from build123d import *

# Parameters (mm, degrees)
CYLINDER_R           = 1.25
CYLINDER_DEPTH       = 2
CYLINDER_PITCH_ANGLE = 90
ARRAY_X_COUNT        = 2
ARRAY_X_PITCH        = 38
ARRAY_Y_COUNT        = 2
ARRAY_Y_PITCH        = 27.5
CYLINDER001_R        = 2
CYLINDER001_DEPTH    = 2
ARRAY001_X_COUNT     = 2
ARRAY001_X_PITCH     = 22
ARRAY001_Y_COUNT     = 2
ARRAY001_Y_PITCH     = 40
BOX001_W             = 2
BOX001_H             = 60
BOX001_DEPTH         = 20
BOX_W                = 40
BOX_H                = 60
BOX_DEPTH            = 2
BOX002_W             = 2
BOX002_H             = 60
BOX002_DEPTH         = 20


with BuildPart() as array:
    # Cylinder → Cylinder (new body)
    with BuildSketch(Plane.XY):
        Circle(CYLINDER_R)
    extrude(amount=CYLINDER_DEPTH)


with BuildPart() as array_1:
    # Cylinder pitch: moved
    add(array.part.rotate(Axis((0, 0, 0), (0, 1, 0)), CYLINDER_PITCH_ANGLE))


with BuildPart() as array_2:
    # Cylinder placement: moved
    add(array_1.part.moved(Location((0, 16.4, 13.5))))

    # Array X: Array ×2


with BuildPart() as array_3:
    add(array_2.part)
    with Locations(*[(i * ARRAY_X_PITCH, 0, 0) for i in range(1, ARRAY_X_COUNT)]):
        add(array_2.part)

    # Array Y: Array ×2


with BuildPart() as array_4:
    add(array_3.part)
    with Locations(*[(0, i * ARRAY_Y_PITCH, 0) for i in range(1, ARRAY_Y_COUNT)]):
        add(array_3.part)


with BuildPart() as array_5:
    # Array placement: moved
    add(array_4.part.moved(Location((2, 40, 0))))


with BuildPart() as array001:
    # Cylinder001 → Cylinder001 (new body)
    with BuildSketch(Plane(origin=(11, 48, 0), x_dir=(1, 0, 0), z_dir=(0, 0, 1))):
        Circle(CYLINDER001_R)
    extrude(amount=CYLINDER001_DEPTH)

    # Array001 X: Array001 ×2


with BuildPart() as array001_1:
    add(array001.part)
    with Locations(*[(i * ARRAY001_X_PITCH, 0, 0) for i in range(1, ARRAY001_X_COUNT)]):
        add(array001.part)

    # Array001 Y: Array001 ×2


with BuildPart() as array001_2:
    add(array001_1.part)
    with Locations(*[(0, i * ARRAY001_Y_PITCH, 0) for i in range(1, ARRAY001_Y_COUNT)]):
        add(array001_1.part)


with BuildPart() as cubo001:
    # Box001 → Box001 (new body)
    with BuildSketch(Plane.XY):
        with Locations((1, 30)):
            Rectangle(BOX001_W, BOX001_H)
    extrude(amount=BOX001_DEPTH)


with BuildPart() as cubo:
    # Box → Box (new body)
    with BuildSketch(Plane.XY):
        with Locations((20, 30)):
            Rectangle(BOX_W, BOX_H)
    extrude(amount=BOX_DEPTH)


with BuildPart() as cut002:
    # Box002 → Box002 (new body)
    with BuildSketch(Plane(origin=(38, 0, 0), x_dir=(1, 0, 0), z_dir=(0, 0, 1))):
        with Locations((1, 30)):
            Rectangle(BOX002_W, BOX002_H)
    extrude(amount=BOX002_DEPTH)

    # Fusion: union Cubo001, Cubo
    add(cubo001.part)
    add(cubo.part)

    # Cut: cut Array
    add(array_5.part, mode=Mode.SUBTRACT)


with BuildPart() as cut002_1:
    # Cut placement: moved
    add(cut002.part.moved(Location((2, 40, 0))))

    # Cut001: cut Array001
    add(array001_2.part, mode=Mode.SUBTRACT)

    # Cut002: cut Array
    add(array_5.part, mode=Mode.SUBTRACT)


solid = cut002_1.part
The listing builds one solid part. Answer for the finished solid, in the listing's coordinates (mm). A direction names the side the tool comes from. Coordinates: 2 decimals unless noted, no trailing zeros. Loops run counter-clockwise (first coordinate to the right, second up) from the corner with the lowest first, then second, coordinate; pieces in that order, holes last.
1) Find section A-A on y = 88. Write down the section's boundary in (x, z).
2) Find the intervals of material crossed by L1, parallel to Y at x = 33, z = 1.15; L2, parallel to X at y = 88, z = 0.7; L3, parallel to X at y = 59.5, z = 12.5, in increasing order.
3) Determine the mould class of faces 1 (the face through (2.99, 55.18, 13.77)), 2 (the face through (21.9, 40, 1.8)), 3 (the face through (3, 70, 20)), 4 (the face through (2.986, 82.791, 12.923)) for opening direction Z: pulls with the +Z half, pulls with the -Z half, needs draft (parallel to the pull), parting line crosses it, or undercut.
4) Find section D-D on y = 56.4. Write down the section's boundary in (x, z), then the cut area to 3 significant figures.
5) A tool of negligible diameter and unlimited length cuts with its end or side. For faces 5 (the face through (41, 70, 20)), 6 (the face through (40, 70, 11)), from which of +Z, -Z, +X, -X, +Y, -Y can it reach the whole face along a straight path? Write none if from no direction.
6) Flat-ended cylindrical pins translate along their axes: pin 1 Ø4.5 at (x, y) = (33, 48) entering from +Z; pin 2 Ø2 at (y, z) = (56.4, 13.5) entering from +X. Find the tip coordinate at first contact, or state that the pin passes through.
7) Find section C-C on x = 33. Write down the section's boundary in (y, z), then the cut area to 3 significant figures.
8) Find section B-B on z = 7.25. Write down the section's boundary in (x, y).
Values:
1. outline: (2, 0) - (9, 0) - (9, 2) - (4, 2) - (4, 20) - (2, 20) - close; (13, 0) - (31, 0) - (31, 2) - (13, 2) - close; (35, 0) - (42, 0) - (42, 20) - (40, 20) - (40, 2) - (35, 2) - close
2. L1: y = 40 to 46, 50 to 86, 90 to 100
2. L2: x = 2 to 9, 13 to 31, 35 to 42
2. L3: x = 2 to 4, 40 to 42
3. face 1: undercut
3. face 2: needs draft
3. face 3: pulls with the +Z half
3. face 4: undercut
4. outline: (2, 0) - (42, 0) - (42, 12.25) - (40, 12.25) - (40, 2) - (4, 2) - (4, 12.25) - (2, 12.25) - close; (2, 14.75) - (4, 14.75) - (4, 20) - (2, 20) - close; (40, 14.75) - (42, 14.75) - (42, 20) - (40, 20) - close
4. area: 142 mm2
5. face 5: +Z, +X, -X, +Y, -Y
5. face 6: +Z, +Y, -Y
6. pin 1: stops at z = 2
6. pin 2: passes through
7. outline: (40, 0) - (46, 0) - (46, 2) - (40, 2) - close; (50, 0) - (86, 0) - (86, 2) - (50, 2) - close; (90, 0) - (100, 0) - (100, 2) - (90, 2) - close
7. area: 104 mm2
8. outline: (2, 40) - (4, 40) - (4, 100) - (2, 100) - close; (40, 40) - (42, 40) - (42, 100) - (40, 100) - close
